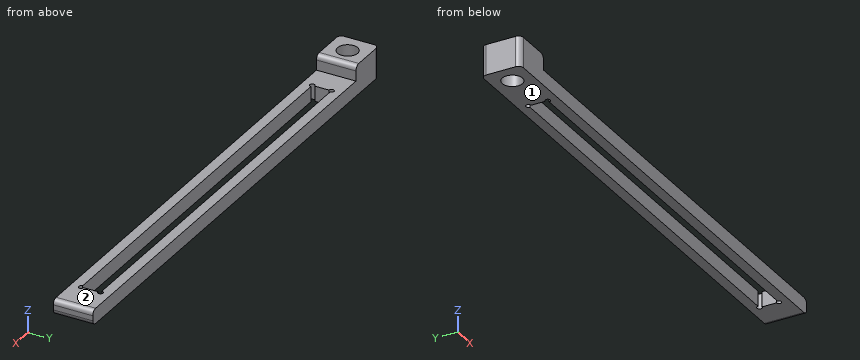
from build123d import *

# Parameters (mm, degrees)
SKIZZE1_W                            = 100
SKIZZE1_H                            = 7.8
SKIZZE1_W_2                          = 80.78
SKIZZE1_H_2                          = 3.8
AUFSATZ_LINEAR_AUSTRAGEN1_DEPTH      = 1.5
SKIZZE3_W                            = 8
SKIZZE3_H                            = 7.8
AUFSATZ_LINEAR_AUSTRAGEN2_DEPTH      = 3
SCHNITT_LINEAR_AUSTRAGEN4_DEPTH      = 51.509504056
SCHNITT_LINEAR_AUSTRAGEN4_DEPTH_BACK = 51.509504056
SKIZZE5_R                            = 2
VERRUNDUNG1_R                        = 1
VERRUNDUNG2_R                        = 1
VERRUNDUNG3_R                        = 1
VERRUNDUNG4_R                        = 1
VERRUNDUNG5_R                        = 1
LOCHUNGSSKIZZE_R                     = 0.5
RAHMENLOCHUNGEN_DEPTH                = 51.241516697


with BuildPart() as part:
    # Skizze1 → Aufsatz-Linear austragen1 (new, symmetric)
    with BuildSketch(Plane.XY):
        Rectangle(SKIZZE1_W, SKIZZE1_H)
        with Locations((3.39, 0)):
            Rectangle(SKIZZE1_W_2, SKIZZE1_H_2, mode=Mode.SUBTRACT)
    extrude(amount=AUFSATZ_LINEAR_AUSTRAGEN1_DEPTH, both=True)

    # Skizze3 → Aufsatz-Linear austragen2 (add)
    with BuildSketch(Plane.XY.offset(1.5)):
        with Locations((-46, 0)):
            Rectangle(SKIZZE3_W, SKIZZE3_H)
    extrude(amount=AUFSATZ_LINEAR_AUSTRAGEN2_DEPTH)

    # Skizze5 → Schnitt-Linear austragen4 (cut, two sides: drawn at the far end of the back side and taken through both)
    with BuildSketch(Plane.XY.offset(4.5).offset(-SCHNITT_LINEAR_AUSTRAGEN4_DEPTH_BACK)):
        with Locations((-46, 0)):
            Circle(SKIZZE5_R)
    extrude(amount=SCHNITT_LINEAR_AUSTRAGEN4_DEPTH + SCHNITT_LINEAR_AUSTRAGEN4_DEPTH_BACK, mode=Mode.SUBTRACT)

    # Verrundung1
    verrundung1_edges = [part.edges().sort_by_distance(p)[0] for p in [
        (-50, 3.9, 1.5),
    ]]
    fillet(verrundung1_edges, radius=VERRUNDUNG1_R)

    # Verrundung2
    verrundung2_edges = [part.edges().sort_by_distance(p)[0] for p in [
        (-50, -3.9, 1.5),
    ]]
    fillet(verrundung2_edges, radius=VERRUNDUNG2_R)

    # Verrundung3
    verrundung3_edges = [part.edges().sort_by_distance(p)[0] for p in [
        (-42, 0, 4.5),
    ]]
    fillet(verrundung3_edges, radius=VERRUNDUNG3_R)

    # Verrundung4
    verrundung4_edges = [part.edges().sort_by_distance(p)[0] for p in [
        (50, 0, -1.5),
    ]]
    fillet(verrundung4_edges, radius=VERRUNDUNG4_R)

    # Verrundung5
    verrundung5_edges = [part.edges().sort_by_distance(p)[0] for p in [
        (50, 0, 1.5),
    ]]
    fillet(verrundung5_edges, radius=VERRUNDUNG5_R)

    # Lochungsskizze → RahmenLochungen (cut, through all)
    with BuildSketch(Plane.XY.offset(1.5)):
        with Locations((-37, 1.9)):
            Circle(LOCHUNGSSKIZZE_R)
        with Locations((-37, -1.9)):
            Circle(LOCHUNGSSKIZZE_R)
        with Locations((43.78, -1.9)):
            Circle(LOCHUNGSSKIZZE_R)
        with Locations((43.78, 1.9)):
            Circle(LOCHUNGSSKIZZE_R)
    extrude(amount=-RAHMENLOCHUNGEN_DEPTH, mode=Mode.SUBTRACT)


solid = part.part
Verification items for the finished model (mm, model axes). Face numbers are marked on the shaded views. A direction names the side the tool comes from. Coordinates: 2 decimals unless noted, no trailing zeros. Order: outer loops, then holes, each group sorted by start corner. A loop starts at its lowest first (then second) coordinate and runs counter-clockwise, first axis right, second up. Notation, with made-up numbers: M 77,77 L 98,77 A24 cw 98,101 Z; hole C 76,-35 d7. An arc over 180 degrees is marked long. Return JSON: item names as keys, results as strings.
1) Access from +Z, -Z, +X, -X, +Y, -Y to the whole of each face (thin tool, end or side, straight path). Record for the marked faces 1 and 2.
Answer list:
{"face 1": "-Z, +X, -X, +Y, -Y", "face 2": "+Z, +X, +Y, -Y"}
2) Cross-section at C-C, the plane z = 2.4. Record the boundary of the cut face in (x, y).
Answer list:
{"outline": "M -50,-2.9 A1 ccw -49,-3.9 L -42,-3.9 L -42,3.9 L -49,3.9 A1 ccw -50,2.9 Z; hole C -46,0 d4"}
3) Thickness scan on L1, parallel to X at y = 0, z = 2.4; L2, parallel to X at y = 2.25, z = 0; L3, parallel to Y at x = -15, z = 1.2. Record the ranges inside material, lowest first. Write a range as [from, to].
Answer list:
{"L1": "[-50, -48], [-44, -42]", "L2": "[-50, -37.36], [-36.64, 43.42], [44.14, 50]", "L3": "[-3.9, -1.9], [1.9, 3.9]"}
4) Cross-section at B-B, the plane x = -15. Record the boundary of the cut face in (y, z).
Answer list:
{"outline": "M -3.9,-1.5 L -1.9,-1.5 L -1.9,1.5 L -3.9,1.5 Z; M 1.9,-1.5 L 3.9,-1.5 L 3.9,1.5 L 1.9,1.5 Z"}
5) Cross-section at D-D, the plane x = -46. Record the boundary of the cut face in (y, z).
Answer list:
{"outline": "M -3.9,-1.5 L -2,-1.5 L -2,4.5 L -3.9,4.5 Z; M 2,-1.5 L 3.9,-1.5 L 3.9,4.5 L 2,4.5 Z"}
6) Gauge pin test, flat ends, axial feed: pin 1 (4 mm diameter, centred on x = -6, y = 0, fed in from +Z); pin 2 (1.6 mm diameter, centred on y = 0, z = 3, fed in from +X); pin 3 (3 mm diameter, centred on x = -46, y = 0, fed in from +Z). Record the tip position at first contact, or that the pin passes through.
Answer list:
{"pin 1": "z = 1.5", "pin 2": "x = -42", "pin 3": "through"}
7) Cross-section at A-A, the plane y = 0. Record the boundary of the cut face in (x, z).
Answer list:
{"outline": "M -50,-1.5 L -48,-1.5 L -48,4.5 L -50,4.5 Z; M -44,-1.5 L -37,-1.5 L -37,1.5 L -42,1.5 L -42,3.5 A1 ccw -43,4.5 L -44,4.5 Z; M 43.78,-1.5 L 49,-1.5 A1 ccw 50,-0.5 L 50,0.5 A1 ccw 49,1.5 L 43.78,1.5 Z"}
